CAD build for the part. Positions are in the model's coordinates, mm. Round coordinates to 2 decimals unless told otherwise and drop trailing zeros. Loops run counter-clockwise (first coordinate to the right, second up) from the corner with the lowest first, then second, coordinate; pieces in that order, holes last.
from build123d import *

# Parameters (mm, degrees)
SWEEP1_PROFILE_R = 2.5


with BuildPart() as part:
    # Sweep1: sweep along a path in Sketch1
    with BuildLine(Plane(origin=(0, 0, 0), x_dir=(1, 0, 0), z_dir=(0, 1, 0))) as sweep1_path:
        Line((-96.132982369, 157.069933949), (88.867017631, 157.069933949))
        ThreePointArc((88.867017631, 157.069933949), (93.463211709, 155.166128026), (95.367017631, 150.569933949))
        Line((95.367017631, 150.569933949), (95.367017631, -139.430066051))
        ThreePointArc((95.367017631, -139.430066051), (93.463211709, -144.026260129), (88.867017631, -145.930066051))
        Line((88.867017631, -145.930066051), (-96.132982369, -145.930066051))
        ThreePointArc((-96.132982369, -145.930066051), (-100.729176446, -144.026260129), (-102.632982369, -139.430066051))
        Line((-102.632982369, -139.430066051), (-102.632982369, 150.569933949))
        ThreePointArc((-102.632982369, 150.569933949), (-100.729176446, 155.166128026), (-96.132982369, 157.069933949))
    # Sweep1 profile (on start of the path) → Sweep1 (sweep)
    with BuildSketch(Plane(origin=(-96.132982369, 0, -157.069933949), x_dir=(0, 0, 1), z_dir=(1, 0, 0))):
        Circle(SWEEP1_PROFILE_R)
    sweep(path=sweep1_path.line)


solid = part.part
Item 1: Cut at A-A (y = 0). List the corners of the cut face in (x, z).
Verdict:
outline: (-105.13, -150.57) arc R9 ccw to (-96.13, -159.57) - (88.87, -159.57) arc R9 ccw to (97.87, -150.57) - (97.87, 139.43) arc R9 ccw to (88.87, 148.43) - (-96.13, 148.43) arc R9 ccw to (-105.13, 139.43) - close; hole (-100.13, -150.57) arc R4 ccw to (-96.13, -154.57) - (88.87, -154.57) arc R4 ccw to (92.87, -150.57) - (92.87, 139.43) arc R4 ccw to (88.87, 143.43) - (-96.13, 143.43) arc R4 ccw to (-100.13, 139.43) - close
Item 2: Flat gauge pin, fed straight in: P1, Ø1, axis at y = 1, z = -50, coming from the +X side. Where does the tip first touch, or does it go through?
Verdict:
P1: stops at x = 97.82
Item 3: Cut at B-B (x = 44). List the corners of the cut face in (y, z), plus the area to 3 significant figures.
Verdict:
outline: circle Ø5 at (0, -157.07); circle Ø5 at (0, 145.93)
area: 39.3 mm2
Item 4: Wall check: L1, parallel to X at y = -0.4, z = -2; L2, parallel to X at y = 0.2, z = -114; L3, parallel to Z at x = -82, y = -0.2. Give the ranges that are in metal, low to high.
Verdict:
L1: x = -105.1 to -100.17, 92.9 to 97.83
L2: x = -105.12 to -100.14, 92.88 to 97.86
L3: z = -159.56 to -154.58, 143.44 to 148.42
Item 5: Cut at C-C (z = 56). List the corners of the cut face in (x, y), plus the area to 3 significant figures.
Verdict:
outline: circle Ø5 at (-102.63, 0); circle Ø5 at (95.37, 0)
area: 39.3 mm2
